The listing builds one solid part. Answer for the finished solid, in the listing's coordinates (mm). Face numbers are marked on the shaded views. A direction names the side the tool comes from. Round coordinates to 2 decimals unless told otherwise and drop trailing zeros. Write each loop counter-clockwise with the first axis right and the second up, starting at its lowest first coordinate (ties: lowest second). Pieces come first, ordered by that corner, then holes.
Item 1: Find the intervals of material crossed by probe 1 along Z at (x, y) = (-14, -13); probe 2 along X at (y, z) = (6.5, 43); probe 3 along Z at (x, y) = (-2, -12.5), in increasing order.
Item 2: Find section D-D on y = -8. Give the vertices of the cut face in (x, z).
Item 3: Find section A-A on x = -2. Give the vertices of the cut face in (y, z), then the cut area to 3 significant figures.
Item 4: Each of these flat-tipped pins is pushed along its axis until it touches: pin 1 (3.5 mm diameter, centred on x = 0.5, z = 32.5, fed in from -Y); pin 2 (18 mm diameter, centred on y = -8, z = 37.5, fed in from +X); pin 3 (4 mm diameter, centred on x = -5, y = -21.5, fed in from +Z); pin 4 (10 mm diameter, centred on x = -8.5, z = 28, fed in from -Y). Where does it stop, or does it pass through?
Item 5: Find section B-B on y = 7. Give the vertices of the cut face in (x, z), then the cut area to 3 significant figures.
Item 6: A tool of negligible diameter and unlimited length cuts with its end or side. For the marked faces 1, 2, 3 and 4, from which of +Z, -Z, +X, -X, +Y, -Y can it reach the whole face along a straight path? Write none if from no direction.
Item 7: Find section C-C on z = 30. Give the vertices of the cut face in (x, y), then the cut area to 3 significant figures.
```python
from build123d import *

# Parameters (mm, degrees)
F0_W     = 45.1892055571
F0_H     = 45.0811590999
F1_DEPTH = 25.4
F2_W     = 12.3209874146
F2_H     = 22.7134097368
F3_DEPTH = 25.4
F4_R     = 12.7


# Not quite as in the source:
# - the program builds the solid bodies; features that only make, move or delete a surface that nothing else refers to are left out


with BuildPart() as f1:
    # F0 (on Top) → F1 (new body)
    with BuildSketch(Plane.XY):
        with Locations((0.0014137477, -4.4078445062)):
            Rectangle(F0_W, F0_H)
    extrude(amount=F1_DEPTH)

    # F2 (on face) → F3 (join)
    with BuildSketch(Plane.XY.offset(25.4)):
        with Locations((1.1841731612, -2.6384368539)):
            Rectangle(F2_W, F2_H)
    extrude(amount=F3_DEPTH)

    # F4
    f4_edges = [f1.edges().sort_by_distance(p)[0] for p in [
        (1.184173, -13.995142, 50.8),
    ]]
    fillet(f4_edges, radius=F4_R)


solid = f1.part
```
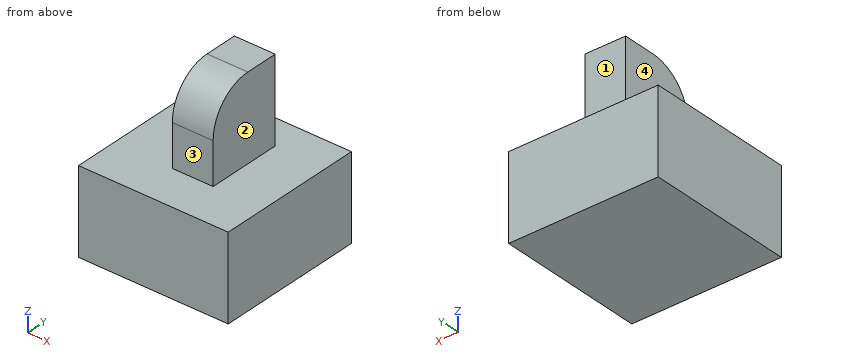
Check values:
1. probe 1: z = 0 to 25.4
1. probe 2: x = -4.98 to 7.34
1. probe 3: z = 0 to 44.08
2. outline: (-22.59, 0) - (22.6, 0) - (22.6, 25.4) - (7.34, 25.4) - (7.34, 48.89) - (-4.98, 48.89) - (-4.98, 25.4) - (-22.59, 25.4) - close
3. outline: (-26.95, 0) - (18.13, 0) - (18.13, 25.4) - (8.72, 25.4) - (8.72, 50.8) - (-1.3, 50.8) arc R12.7 ccw to (-14, 38.1) - (-14, 25.4) - (-26.95, 25.4) - close
3. area: 1,690 mm2
4. pin 1: stops at y = -14
4. pin 2: stops at x = 7.34
4. pin 3: stops at z = 25.4
4. pin 4: stops at y = -26.95
5. outline: (-22.59, 0) - (22.6, 0) - (22.6, 25.4) - (7.34, 25.4) - (7.34, 50.8) - (-4.98, 50.8) - (-4.98, 25.4) - (-22.59, 25.4) - close
5. area: 1,460 mm2
6. face 1: +Z, +X, -X, +Y
6. face 2: +Z, +X, +Y, -Y
6. face 3: +Z, +X, -X, -Y
6. face 4: +Z, -X, +Y, -Y
7. outline: (-4.98, -14) - (7.34, -14) - (7.34, 8.72) - (-4.98, 8.72) - close
7. area: 280 mm2
